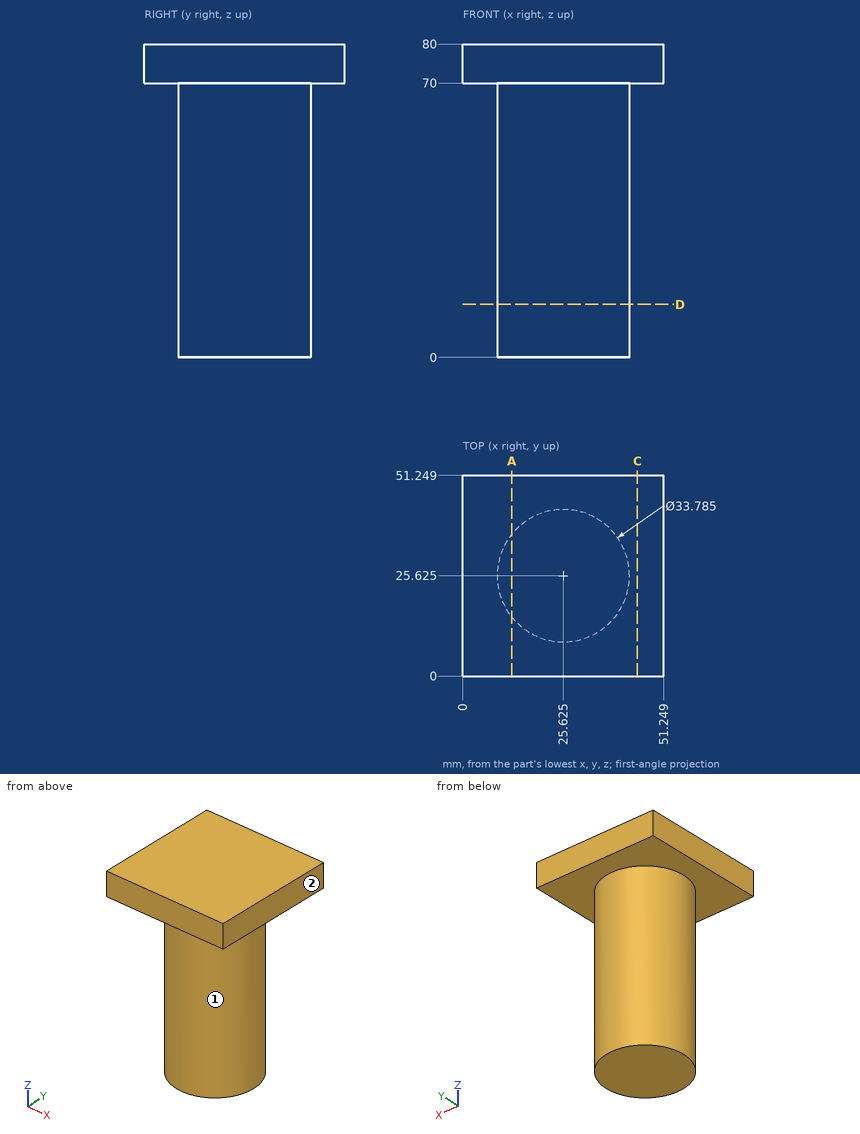
Design review of the part shown in the three views and the two pictorial views. Dimensions are in mm from the part's minimum x, y and z. A direction names the side the tool comes from. Round coordinates to 2 decimals unless told otherwise and drop trailing zeros. Loops run counter-clockwise (first coordinate to the right, second up) from the corner with the lowest first, then second, coordinate; pieces in that order, holes last. Notation, with made-up numbers: M -13.75,88 L 6.25,88 A22 cw 6.25,118 Z; hole C 35,4 d3. An arc over 180 degrees is marked long. Answer as a JSON object with one key per item and string values.
Item 1: Clearance check with flat-ended pins moving along their axes: P1, Ø1.5, axis at x = 37, z = 42, coming from the -Y side; P2, Ø6, axis at y = 22, z = 28, coming from the +X side (1 decimal); P3, Ø6, axis at x = 5.5, y = 14.5, coming from the -Z side. State where each tip first meets the part, or that it passes through.
Check sheet entries:
{"P1": "y = 12.49", "P2": "x = 42.5", "P3": "z = 70"}
Item 2: We need section A-A, the plane x = 12.5. State the section outline as (y, z) points, and give its area (3 significant figures).
Check sheet entries:
{"outline": "M 0,70 L 14.99,70 L 14.99,0 L 36.26,0 L 36.26,70 L 51.25,70 L 51.25,80 L 0,80 Z", "area": "2,000 mm2"}
Item 3: We need section C-C, the plane x = 44.5. State the section outline as (y, z) points.
Check sheet entries:
{"outline": "M 0,70 L 51.25,70 L 51.25,80 L 0,80 Z"}
Item 4: For line 1 along Z through (x, y) = (41.5, 9); line 2 along X through (y, z) = (38, 32.5) (1 decimal); line 3 along X through (y, z) = (14, 69), list the stretches that pass through material, from the lowest coordinate up.
Check sheet entries:
{"line 1": "70 to 80", "line 2": "14.1 to 37.1", "line 3": "13.37 to 37.88"}
Item 5: Tool access review of the marked faces 1 and 2: name each direction out of +Z, -Z, +X, -X, +Y, -Y from which nothing blocks a thin tool from reaching the whole face with its end or side.
Check sheet entries:
{"face 1": "-Z", "face 2": "+Z, -Z, +X, +Y, -Y"}
Item 6: We need section D-D, the plane z = 13.5. State the section outline as (x, y) points (1 decimal).
Check sheet entries:
{"outline": "C 25.6,25.6 d33.8"}
